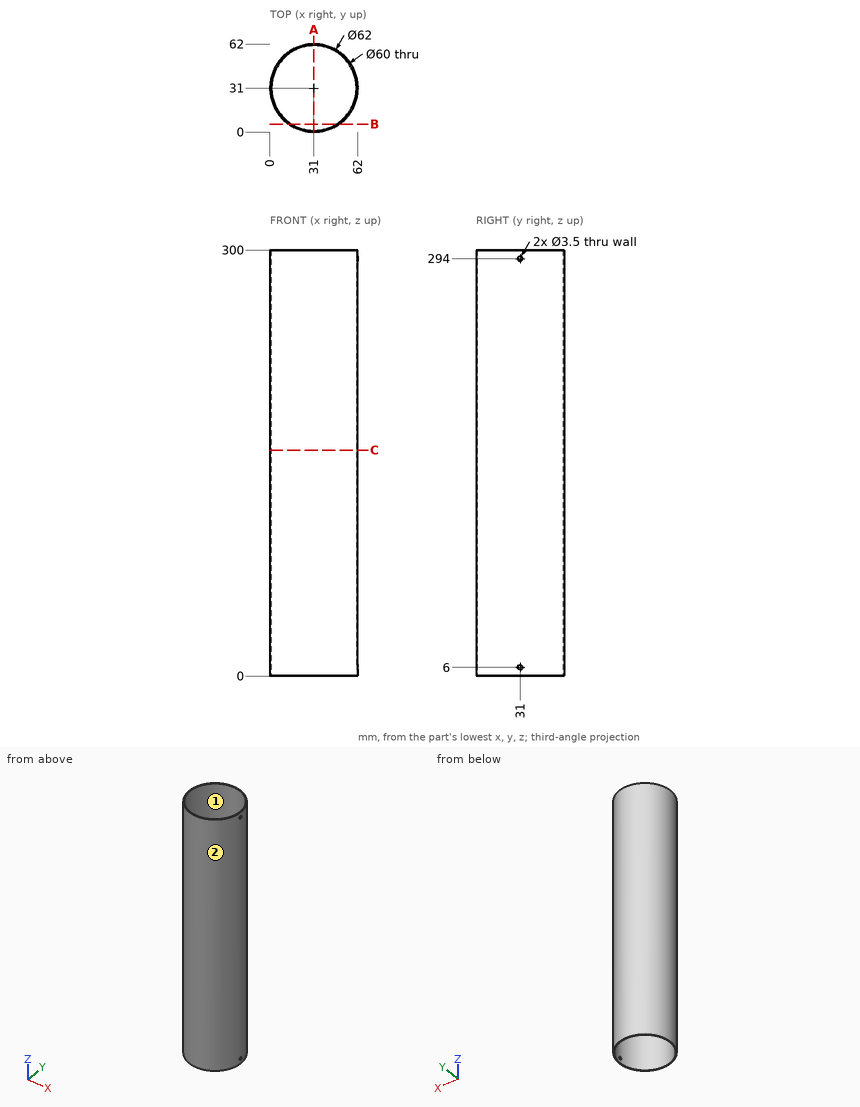
Geometry check sheet. Reference: drawing and pictorial views, mm from the part's lowest x, y, z. Round coordinates to 2 decimals unless told otherwise and drop trailing zeros. Write each loop counter-clockwise with the first axis right and the second up, starting at its lowest first coordinate (ties: lowest second). Pieces come first, ordered by that corner, then holes. Notation, with made-up numbers: (37.5, -0.5) -> (81.5, -0.5) arc R10 ccw to (81.5, 5.5) -> close; hole circle Ø8 at (-40, -27). An arc over 180 degrees is marked (long way). Put each result on its own line as item: value.
1) Cross-section at B-B, the plane y = 5.5. Enter the section's corners in (x, z), plus the area to 3 significant figures.
Recorded:
outline: (13.37, 0) -> (15.2, 0) -> (15.2, 300) -> (13.37, 300) -> close; (46.8, 0) -> (48.63, 0) -> (48.63, 300) -> (46.8, 300) -> close
area: 1,090 mm2
2) Depth check by flat-ended pin: P1, Ø12, axis at y = 51, z = 132, coming from the -X side; P2, Ø1, axis at x = 25, z = 135, coming from the -Y side; P3, Ø12, axis at y = 7, z = 45, coming from the +X side; P4, Ø4.5, axis at y = 31, z = 294, coming from the +X side. Enter the tip coordinate at first touch or a pass-through.
Recorded:
P1: stops at x = 3.34
P2: stops at y = 0.49
P3: stops at x = 56.24
P4: stops at x = 62
3) Cross-section at A-A, the plane x = 31. Enter the section's corners in (y, z).
Recorded:
outline: (0, 0) -> (1, 0) -> (1, 300) -> (0, 300) -> close; (61, 0) -> (62, 0) -> (62, 300) -> (61, 300) -> close
4) Cross-section at C-C, the plane z = 159. Enter the section's corners in (x, y).
Recorded:
outline: circle Ø62 at (31, 31); hole circle Ø60 at (31, 31)
5) Thickness scan on probe 1 along Y at (x, z) = (31, 143); probe 2 along X at (y, z) = (54, 191); probe 3 along Y at (x, z) = (45.5, 176). Record the ranges inside material, lowest first. Write a range as from..to.
Recorded:
probe 1: y = 0..1, 61..62
probe 2: x = 10.22..11.74, 50.26..51.78
probe 3: y = 3.6..4.74, 57.26..58.4
6) Release check for a two-part mould opening along X. For the marked faces 1 and 2 record: pulls with the +X half, pulls with the -X half, needs draft (parallel to the pull), parting line crosses it, or undercut.
Recorded:
face 1: undercut
face 2: parting line crosses it
